The drawing under review shows one solid part. Ordinate dimensions are in mm from its lowest x, y, z. Give positions to 0.01 mm unless a question says otherwise; leave off trailing zeros. Order: outer loops, then holes, each group sorted by start corner. A loop starts at its lowest first (then second) coordinate and runs counter-clockwise, first axis right, second up. Notation, with made-up numbers: (47.25, -33) - (64.25, -33) arc R24 ccw to (64.25, 5) - close; hole circle Ø8 at (19, 3.25). An arc over 180 degrees is marked (long way). Answer as a JSON object with one key per item and string values. Group by question number.
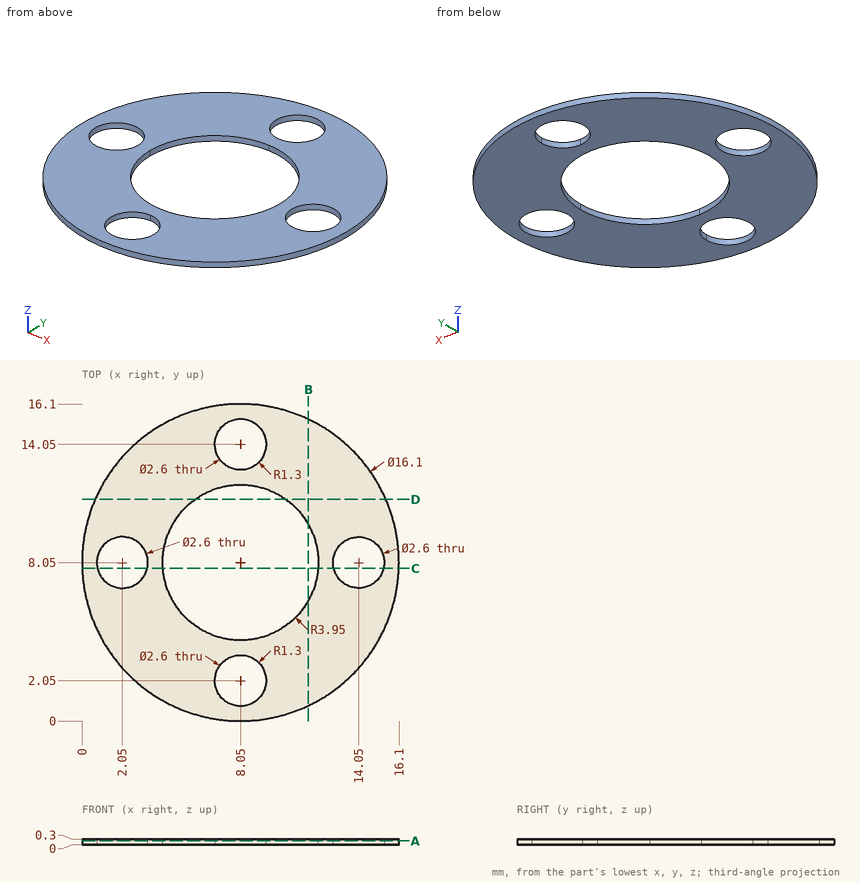
1) For line 1 (Y direction, x = 8.05, z = 0.25); line 2 (X direction, y = 8.5, z = 0.1); line 3 (X direction, y = 13.5, z = 0.1), list the stretches that pass through material, from the lowest coordinate up.
2) Consider section C-C (y = 7.75). Give the boundary of the cut face in (x, z).
3) Consider section B-B (x = 11.5). Give the boundary of the cut face in (y, z).
4) Consider section A-A (z = 0.2). Give the boundary of the cut face in (x, y).
5) Consider section D-D (y = 11.25). Give the boundary of the cut face in (x, z), plus the area to 3 significant figures.
Result set:
{
 "1": {"line 1": "y = 0 to 0.75, 3.35 to 4.1, 12 to 12.75, 15.35 to 16.1", "line 2": "x = 0.01 to 0.83, 3.27 to 4.13, 11.97 to 12.83, 15.27 to 16.09", "line 3": "x = 2.13 to 6.87, 9.23 to 13.97"},
 "2": {"outline": "(0.01, 0) - (0.79, 0) - (0.79, 0.3) - (0.01, 0.3) - close; (3.31, 0) - (4.11, 0) - (4.11, 0.3) - (3.31, 0.3) - close; (11.99, 0) - (12.79, 0) - (12.79, 0.3) - (11.99, 0.3) - close; (15.31, 0) - (16.09, 0) - (16.09, 0.3) - (15.31, 0.3) - close"},
 "3": {"outline": "(0.78, 0) - (6.13, 0) - (6.13, 0.3) - (0.78, 0.3) - close; (9.97, 0) - (15.32, 0) - (15.32, 0.3) - (9.97, 0.3) - close"},
 "4": {"outline": "circle Ø16.1 at (8.05, 8.05); hole circle Ø2.6 at (2.05, 8.05); hole (4.1, 8.05) arc R3.95 ccw to (8.05, 4.1) arc R3.95 ccw to (12, 8.05) arc R3.95 ccw to (8.05, 12) arc R3.95 ccw to start; hole circle Ø2.6 at (8.05, 2.05); hole circle Ø2.6 at (8.05, 14.05); hole circle Ø2.6 at (14.05, 8.05)"},
 "5": {"outline": "(0.66, 0) - (5.73, 0) - (5.73, 0.3) - (0.66, 0.3) - close; (10.37, 0) - (15.44, 0) - (15.44, 0.3) - (10.37, 0.3) - close", "area": "3.04 mm2"}
}
